Could you check a few things on this model? Use its own coordinates, in mm. A direction names the side the tool comes from. Give positions to 0.01 mm unless a question says otherwise; leave off trailing zeros. Order: outer loops, then holes, each group sorted by start corner. A loop starts at its lowest first (then second) coordinate and runs counter-clockwise, first axis right, second up. Notation, with made-up numbers: (43, 86) -> (93, 86) arc R17 cw to (93, 110) -> close; hole circle Ø6 at (65.5, 34.25). An arc over 180 degrees is marked (long way). Answer as CSV lines item,"result". Start each with the question number.
(1) I want a section at C-C (y = 2.75). Please give me the cut outline in (x, z).
(2) I want a section at A-A (z = 1.7). Please give me the cut outline in (x, y), plus the area to 3 significant figures.
(3) Will these pins go through, and if not, where does the flat tip stop? pin 1 Ø3 at (y, z) = (-2.5, 3) entering from +X; pin 2 Ø2 at (y, z) = (-0.5, 3.5) entering from +X.
(4) On a 3-axis mill with a long thin cutter (end or side, diameter ignored), from which of +Z, -Z, +X, -X, +Y, -Y can I reach the whole of each face in a straight line? I mean faces 4 (the face through (-36, 0, 5)), 5 (the face through (-56, -4, 2)). Say none if no direction works.
(5) I want a section at B-B (y = -1.75). Please give me the cut outline in (x, z).
(6) I need wall thicknesses on L1, parallel to X at y = 0, z = 3; L2, parallel to Y at x = -54.5, z = 4.85; L3, parallel to X at y = 2.25, z = 4.85. Which ranges of each line are inside material? Lowest first, please.
(7) We'd pull the mould along X, two halves only. Please class faces 1 (the face through (-38, -7.5, 2)), 2 (the face through (-60.9, 6.93, 2.54)), 3 (the face through (-53.5, 0, 2)): released by +X, released by -X, zero draft, split by the parting line, or undercut.
Autodesk Inventor part; units mm, degrees
ref_plane "YZ Plane" through (0, 0, 0) normal (1, 0, 0) x (0, 1, 0)
ref_plane "XZ Plane" through (0, 0, 0) normal (0, 1, 0) x (-1, 0, 0)
ref_plane "XY Plane" through (0, 0, 0) normal (0, 0, 1) x (1, 0, 0)
sketch "Skizze1" plane through (0, 0, 0) normal (0, 0, 1) x (1, 0, 0)
  line L0 (0, -24.15) -> (0, 24.15)
  line L1 (-77.25, 0) -> (33, 0)
  circle A0 centre (-15.5, 15.5) radius 1.75
  circle A1 centre (15.5, 15.5) radius 1.75
  circle A2 centre (-15.5, -15.5) radius 1.75
  circle A3 centre (15.5, -15.5) radius 1.75
  circle A4 centre (-16.5, 0) radius 11
  circle A5 centre (0, 0) radius 5.5
  circle A6 centre (-16.5, 0) radius 4
  arc A7 (-16.5, -7.5) -> (-16.5, 7.5) centre (-16.5, 0) ccw
  line L2 (-16.5, 7.5) -> (-36.5, 7.5)
  line L3 (-36.5, 7.5) -> (-61.5, 7.5)
  line L4 (-61.5, 7.5) -> (-61.5, -7.5)
  line L5 (-61.5, -7.5) -> (-16.5, -7.5)
  dimension "d0" = 3.5
  dimension "d1" = 15.5
  dimension "d2" = 15.5
  dimension "d3" = 22
  dimension "d4" = 16.5
  dimension "d5" = 11
  dimension "d6" = 8
  dimension "d7" = 15
  dimension "d10" = 15
  dimension "d11" = 45
extrude "Extrusion1" add sketch "Skizze1" along normal blind 5 contours A7 L5 A4 L1 A6 | L1 A6 A4 L2 A7 | A4 L1 L4 L3 L2 | L5 L4 L1 A4
sketch "Skizze3" plane through (0, 0, 0) normal (0, 0, -1) x (-1, 0, 0)
  circle A0 centre (16.5, 0) radius 4
  arc A1 (16.5, 7.5) -> (16.5, -7.5) centre (16.5, 0) ccw
  line L0 (16.5, -7.5) -> (61.5, -7.5)
  line L1 (61.5, -7.5) -> (61.5, 7.5)
  line L2 (61.5, 7.5) -> (16.5, 7.5)
  line L3 (58.5, -4) -> (53.5, -4)
  line L4 (53.5, -4) -> (53.5, 4)
  line L5 (53.5, 4) -> (58.5, 4)
  line L6 (58.5, 4) -> (58.5, -4)
  line L7 (73.8, 0) -> (-12.3, 0)
  point P0 (0, 0)
  dimension "d17" = 5
  dimension "d18" = 8
  dimension "d19" = 3
extrude "Extrusion3" cut sketch "Skizze3" against normal blind 5 contours L7 L6 L3 L4 | L4 L5 L6 L7
fillet "Rundung1" radius 2 2 edges at (-61.5, -7.5, 2.5) (-61.5, 7.5, 2.5)
properties part number "Kugellager-Schieber-Seite" material "ABS-Kunststoff"
Final values:
1,outline,"(-61.5, 0) -> (-58.5, 0) -> (-58.5, 5) -> (-61.5, 5) -> close; (-53.5, 0) -> (-19.4, 0) -> (-19.4, 5) -> (-53.5, 5) -> close; (-13.6, 0) -> (-9.52, 0) -> (-9.52, 5) -> (-13.6, 5) -> close"
2,outline,"(-61.5, -5.5) arc R2 ccw to (-59.5, -7.5) -> (-16.5, -7.5) arc R7.5 ccw to (-16.5, 7.5) -> (-59.5, 7.5) arc R2 ccw to (-61.5, 5.5) -> close; hole (-58.5, -4) -> (-53.5, -4) -> (-53.5, 4) -> (-58.5, 4) -> close; hole circle Ø8 at (-16.5, 0)"
2,area,"671 mm²"
3,pin 1,"x = -9.07"
3,pin 2,"x = -9"
4,face 4,"+Z, +X, -X, +Y, -Y"
4,face 5,"+Z, -Z"
5,outline,"(-61.5, 0) -> (-58.5, 0) -> (-58.5, 5) -> (-61.5, 5) -> close; (-53.5, 0) -> (-20.1, 0) -> (-20.1, 5) -> (-53.5, 5) -> close; (-12.9, 0) -> (-9.21, 0) -> (-9.21, 5) -> (-12.9, 5) -> close"
6,L1,"-61.5 to -58.5, -53.5 to -20.5, -12.5 to -9"
6,L2,"-7.5 to -4, 4 to 7.5"
6,L3,"-61.5 to -58.5, -53.5 to -19.81, -13.19 to -9.35"
7,face 1,"zero draft"
7,face 2,"released by -X"
7,face 3,"undercut"
